from build123d import *

# Parameters (mm, degrees)
SKETCH_1_R           = 18
EXTRUDE_1_DEPTH      = 2
SKETCH_2_W           = 2
SKETCH_2_H           = 30
EXTRUDE_2_DEPTH      = 15
HOLE_WIZARD_M3_5_1_D = 2.9
SKETCH_6_R           = 17
CUT_EXTRUDE_1_DEPTH  = 15


with BuildPart() as part:
    # 草图1 → 凸台-拉伸1 (new body)
    with BuildSketch(Plane(origin=(0, 0, 0), x_dir=(1, 0, 0), z_dir=(0, 1, 0))):
        Circle(SKETCH_1_R)
        with BuildLine():
            Line((-9.949874371, 15), (-52, 15))
            Line((-52, 15), (-52, -15))
            Line((-52, -15), (-9.949874371, -15))
            ThreePointArc((-9.949874371, -15), (-18, 0), (-9.949874371, 15))
        make_face()
    extrude(amount=EXTRUDE_1_DEPTH)

    # 草图2 → 凸台-拉伸2 (add)
    with BuildSketch(Plane(origin=(0, 2, 0), x_dir=(1, 0, 0), z_dir=(0, 1, 0))):
        with Locations((-51, 0)):
            Rectangle(SKETCH_2_W, SKETCH_2_H)
    extrude(amount=EXTRUDE_2_DEPTH)

    # M3.5 螺纹孔1 (through all)
    with Locations(Plane(origin=(-50, 0, 0), x_dir=(0, 0, -1), z_dir=(1, 0, 0))):
        with Locations((-8, 9.5), (8, 9.5)):
            Hole(HOLE_WIZARD_M3_5_1_D / 2)

    # 草图6 → 切除-拉伸1 (cut)
    with BuildSketch(Plane(origin=(0, 2, 0), x_dir=(1, 0, 0), z_dir=(0, 1, 0))):
        with Locations(Location((0, 0, 0), (0, 0, 270))):
            Circle(SKETCH_6_R)
    extrude(amount=-CUT_EXTRUDE_1_DEPTH, mode=Mode.SUBTRACT)


solid = part.part
Build history of the part. All positions in model axes, mm. A direction names the side the tool comes from. Round coordinates to 2 decimals unless told otherwise and drop trailing zeros. Loops run counter-clockwise (first coordinate to the right, second up) from the corner with the lowest first, then second, coordinate; pieces in that order, holes last. Notation, with made-up numbers: (-39.75, -38) -> (-11.75, -38) arc R22 ccw to (-11.75, -12) -> close; hole circle Ø10 at (43.5, -24.5). An arc over 180 degrees is marked (long way). One line per item, written item: value. Start each with the question number.
Q1. Cut at A-A on y = 9.5. List the corners of the cut face in (x, z).
Q2. Probe line 1 along X through (y, z) = (16, 6); line 2 along Y through (x, z) = (-50.95, -8); line 3 along Z through (x, y) = (2.5, 1.75). List the from-to ranges inside material, lowest first.
Q3. Cut at C-C on z = -2. List the corners of the cut face in (x, y).
Q4. Drop flat-ended pins along their axis: pin 1 Ø18 at (x, z) = (-19, -6.5) entering from +Y; pin 2 Ø7.5 at (y, z) = (9, -0.5) entering from +X; pin 3 Ø3 at (y, z) = (3, -9) entering from +X. Give the stop position or say it passes through.
Q5. Two-plate mould, pull along Y, no slides. Class faces 4 (the face through (-51.01, 8.62, 6.85)), 5 (the face through (-50, 9, 0)), 6 (the face through (-32, 2, 0)): released by +Y, released by -Y, zero draft, split by the parting line, or undercut.
Q6. Cut at B-B on x = 0. List the corners of the cut face in (y, z).
Q7. 3-axis set-ups, long thin cutter, end or side, ignore diameter. For faces 1 (the face through (-35.7, 1.5, -15)), 2 (the face through (16.855, 1.014, -2.213)), 3 (the face through (-35.7, 1.5, 15)): which of +Z, -Z, +X, -X, +Y, -Y reach the whole face in a straight line?
Q8. Cut at D-D on z = 8. List the corners of the cut face in (x, y).
Computed:
1. outline: (-52, -15) -> (-50, -15) -> (-50, -9.45) -> (-52, -9.45) -> close; (-52, -6.55) -> (-50, -6.55) -> (-50, 6.55) -> (-52, 6.55) -> close; (-52, 9.45) -> (-50, 9.45) -> (-50, 15) -> (-52, 15) -> close
2. line 1: -52 to -50
2. line 2: 0 to 8.05, 10.95 to 17
2. line 3: -17.83 to -16.82, 16.82 to 17.83
3. outline: (-52, 0) -> (-16.88, 0) -> (-16.88, 2) -> (-50, 2) -> (-50, 17) -> (-52, 17) -> close; (16.88, 0) -> (17.89, 0) -> (17.89, 2) -> (16.88, 2) -> close
4. pin 1: y = 2
4. pin 2: x = -50
4. pin 3: x = 16.18
5. face 4: undercut
5. face 5: zero draft
5. face 6: released by +Y
6. outline: (0, -18) -> (2, -18) -> (2, -17) -> (0, -17) -> close; (0, 17) -> (2, 17) -> (2, 18) -> (0, 18) -> close
7. face 1: -Z, -X, +Y, -Y
7. face 2: +Y, -Y
7. face 3: +Z, -X, +Y, -Y
8. outline: (-52, 0) -> (-15, 0) -> (-15, 2) -> (-50, 2) -> (-50, 8.05) -> (-52, 8.05) -> close; (-52, 10.95) -> (-50, 10.95) -> (-50, 17) -> (-52, 17) -> close; (15, 0) -> (16.12, 0) -> (16.12, 2) -> (15, 2) -> close
